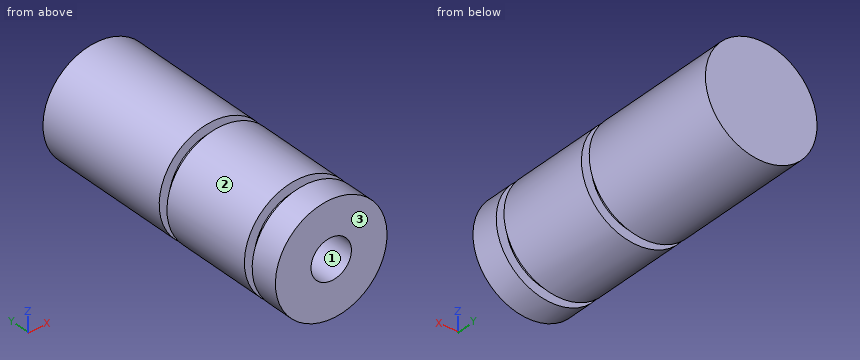
from build123d import *

# Parameters (mm, degrees)
SKETCH1_R           = 5.8
BOSS_EXTRUDE1_DEPTH = 30
SKETCH2_R           = 2.1
CUT_EXTRUDE1_DEPTH  = 10
SKETCH3_R           = 5.8
SKETCH3_R_2         = 4.8
CUT_EXTRUDE2_DEPTH  = 1
CUT_EXTRUDE3_START  = 1
SKETCH4_R           = 5.8
SKETCH4_R_2         = 4.8
CUT_EXTRUDE3_DEPTH  = 1


with BuildPart() as part:
    # Sketch1 → Boss-Extrude1 (new body)
    with BuildSketch(Plane(origin=(0, 0, 0), x_dir=(1, 0, 0), z_dir=(0, 1, 0))):
        with Locations(Location((0, 0, 0), (0, 0, 270))):
            Circle(SKETCH1_R)
    extrude(amount=BOSS_EXTRUDE1_DEPTH)

    # Sketch2 → Cut-Extrude1 (cut)
    with BuildSketch(Plane.XZ):
        with Locations(Location((0, 0, 0), (0, 0, 270))):
            Circle(SKETCH2_R)
    extrude(amount=-CUT_EXTRUDE1_DEPTH, mode=Mode.SUBTRACT)

    # Sketch3 → Cut-Extrude2 (cut)
    with BuildSketch(Plane(origin=(0, 14, 0), x_dir=(-1, 0, 0), z_dir=(0, -1, 0))):
        with Locations(Location((0, 0, 0), (0, 0, 90))):
            Circle(SKETCH3_R)
        with Locations(Location((0, 0, 0), (0, 0, 90))):
            Circle(SKETCH3_R_2, mode=Mode.SUBTRACT)
    extrude(amount=-CUT_EXTRUDE2_DEPTH, mode=Mode.SUBTRACT)

    # Sketch4 → Cut-Extrude3 (cut)
    with BuildSketch(Plane(origin=(0, 4, 0), x_dir=(-1, 0, 0), z_dir=(0, -1, 0)).offset(CUT_EXTRUDE3_START)):
        with Locations(Location((0, 0, 0), (0, 0, 90))):
            Circle(SKETCH4_R)
        with Locations(Location((0, 0, 0), (0, 0, 90))):
            Circle(SKETCH4_R_2, mode=Mode.SUBTRACT)
    extrude(amount=-CUT_EXTRUDE3_DEPTH, mode=Mode.SUBTRACT)


solid = part.part
Read the model definition and answer for the solid it produces. Units are mm, in the model's axes. Face numbers are marked on the shaded views. Coordinates: 2 decimals unless noted, no trailing zeros. Write each loop counter-clockwise with the first axis right and the second up, starting at its lowest first coordinate (ties: lowest second). Pieces come first, ordered by that corner, then holes. Notation, with made-up numbers: (51.5, 59.5) - (75.5, 59.5) arc R18 cw to (75.5, 92.5) - close; hole circle Ø1 at (37.5, 22). An arc over 180 degrees is marked (long way). One line per question, with ' | ' between items.
Q1. Each of these flat-tipped pins is pushed along its axis until it touches: P1, Ø6, axis at y = 15, z = 2.5, coming from the -X side; P2, Ø1.5, axis at y = 10.5, z = -2, coming from the +X side; P3, Ø1.3, axis at x = 1, z = -0.5, coming from the -Y side; P4, Ø1, axis at y = 25.5, z = -2, coming from the +X side. Where does it stop, or does it pass through?
Result set:
P1: x = -5.8 | P2: x = 5.66 | P3: y = 10 | P4: x = 5.6
Q2. Determine the mould class of the marked faces 1, 2 and 3 for opening direction X: +X half, -X half, draft (parallel to the pull), parting line (faces both ways), or undercut.
Result set:
face 1: undercut | face 2: parting line | face 3: draft
Q3. Find section B-B, the plane z = 0. Write down the section's boundary in (x, y).
Result set:
outline: (-5.8, 0) - (-2.1, 0) - (-2.1, 10) - (2.1, 10) - (2.1, 0) - (5.8, 0) - (5.8, 3) - (4.8, 3) - (4.8, 4) - (5.8, 4) - (5.8, 14) - (4.8, 14) - (4.8, 15) - (5.8, 15) - (5.8, 30) - (-5.8, 30) - (-5.8, 15) - (-4.8, 15) - (-4.8, 14) - (-5.8, 14) - (-5.8, 4) - (-4.8, 4) - (-4.8, 3) - (-5.8, 3) - close
Q4. Find section A-A, the plane x = 0. Write down the section's boundary in (y, z), plus the area to 3 significant figures.
Result set:
outline: (0, -5.8) - (3, -5.8) - (3, -4.8) - (4, -4.8) - (4, -5.8) - (14, -5.8) - (14, -4.8) - (15, -4.8) - (15, -5.8) - (30, -5.8) - (30, 5.8) - (15, 5.8) - (15, 4.8) - (14, 4.8) - (14, 5.8) - (4, 5.8) - (4, 4.8) - (3, 4.8) - (3, 5.8) - (0, 5.8) - (0, 2.1) - (10, 2.1) - (10, -2.1) - (0, -2.1) - close | area: 302 mm^2
Q5. Find section C-C, the plane y = 4.75. Write down the section's boundary in (x, z).
Result set:
outline: circle Ø11.6 at (0, 0); hole circle Ø4.2 at (0, 0)
Q6. Find section D-D, the plane z = 4.5. Write down the section's boundary in (x, y).
Result set:
outline: (-3.66, 0) - (3.66, 0) - (3.66, 3) - (1.67, 3) - (1.67, 4) - (3.66, 4) - (3.66, 14) - (1.67, 14) - (1.67, 15) - (3.66, 15) - (3.66, 30) - (-3.66, 30) - (-3.66, 15) - (-1.67, 15) - (-1.67, 14) - (-3.66, 14) - (-3.66, 4) - (-1.67, 4) - (-1.67, 3) - (-3.66, 3) - close
Q7. Consider L1, parallel to Y at x = 5, z = 0; L2, parallel to X at y = 5.5, z = 0; L3, parallel to Y at x = 0.5, z = 1. Determine where each line is inside the solid, lowest interval first. Write a range as [from, to].
Result set:
L1: [0, 3], [4, 14], [15, 30] | L2: [-5.8, -2.1], [2.1, 5.8] | L3: [10, 30]
